Autodesk Inventor part; units mm, degrees
ref_plane "YZ Plane" through (0, 0, 0) normal (1, 0, 0) x (0, 1, 0)
ref_plane "XZ Plane" through (0, 0, 0) normal (0, 1, 0) x (-1, 0, 0)
ref_plane "XY Plane" through (0, 0, 0) normal (0, 0, 1) x (1, 0, 0)
sketch "Sketch1" plane through (0, 0, 0) normal (0, 0, 1) x (1, 0, 0)
  line L0 (17.5514, 0) -> (46.0756, 0)
  line L1 (46.0756, 0) -> (46.0756, 12.7)
  line L2 (46.0756, 12.7) -> (0, 12.7)
  line L3 (0, 12.7) -> (0, 0)
  line L4 (17.5514, 12.7) -> (17.5514, 0)
  line L5 (46.0756, 8.9662) -> (42.3672, 8.9662)
  line L6 (42.3672, 7.747) -> (42.3672, 0)
  line L7 (46.0756, 7.747) -> (42.3672, 7.747)
  line L8 (46.0756, 8.9662) -> (42.3672, 7.747)
  line L9 (0, 11.1252) -> (0, 12.7)
  line L10 (17.5514, 0) -> (23.85, 0)
  line L11 (0, -2.5) -> (0, 0)
  line L12 (0, 12.7) -> (38.0365, 12.7)
  line L13 (38.0365, 12.7) -> (38.0365, 14.2748)
  line L14 (38.0365, 14.2748) -> (0, 14.2748)
  line L15 (0, 14.2748) -> (0, 12.7)
  line L16 (17.5514, 12.7) -> (17.5514, 14.2748)
  line L17 (0, 0) -> (17.5514, 0)
  line L18 (0, 14.2748) -> (10.6426, 14.2748)
  line L19 (10.6426, 14.2748) -> (10.6426, 26.2128)
  line L20 (10.6426, 26.2128) -> (0, 26.2128)
  line L21 (0, 26.2128) -> (0, 14.2748)
  dimension "d1" = 12.7
  dimension "d3" = 3.7338
  dimension "d5" = 4.953
  dimension "d8" = 17.5514
  dimension "d9" = 42.3672
  dimension "d10" = 46.0756
  dimension "d11" = 1.5748
  dimension "d12" = 38.0365
  dimension "d23" = 11.938
  dimension "d24" = 10.6426
revolve "Revolution1" add sketch "Sketch1" angle 360 about axis through (0, 12.7, 0) along (0, -1, 0) contours L4 L2 L1 L8 L6 L0 | L17 L3 L2 L4 | L16 L14 L13 L2 | L2 L15 L14 L16 | L21 L20 L19 L14
sketch "Sketch2" plane through (0, 14.2748, 0) normal (0, 1, 0) x (1, 0, 0)
  circle A0 centre (0, 0) radius 30.1752
  point P0 (0, 30.1752)
  point P1 (0, -30.1752)
  dimension "d14" = 60.3504
hole "Hole1" at (0, 14.2748, -30.1752) at (0, 14.2748, 30.1752) direction (0, -1, 0) diameter 6.35 depth 7.62
fillet "Fillet1" radius 3.175 1 edges at (-42.3672, 0, 0)
sketch "Sketch3" plane through (0, 26.2128, 0) normal (0, 1, 0) x (1, 0, 0)
  point P0 (0, 0)
  point P1 (0, 0)
hole "Hole2" at (0, 26.2128, 0) direction (0, -1, 0) diameter 12.9794 end through all
chamfer "Chamfer1" distance 1.27 angle 45 1 edges at (0, 0, -6.4897)
chamfer "Chamfer2" distance 1.27 angle 45 1 edges at (-10.6426, 26.2128, 0)
properties part number "2016.06.09 ThorLabs Photodiode Adapter" material "Aluminum 6061"
CAD build for the part. Positions are in the model's coordinates, mm. A direction names the side the tool comes from. Give positions to 0.01 mm unless a question says otherwise; leave off trailing zeros. Write each question's results on one line, items separated by ' | '.
Q1. Probe probe 1 along Z at (x, y) = (0, 12.5); probe 2 along Z at (x, y) = (0, 16.25); probe 3 along Y at (x, z) = (2, 18). List the from-to ranges inside material, lowest first.
Geometry check:
probe 1: z = -46.08 to -33.35, -27 to -6.49, 6.49 to 27, 33.35 to 46.08 | probe 2: z = -10.64 to -6.49, 6.49 to 10.64 | probe 3: y = 0 to 14.27
Q2. Mould opens along X. For faces 3 (the face through (-0.954, 10.411, 33.204)), 4 (the face through (-9.18, 5.43, -41.36)), 5 (the face through (0, 6.655, 30)), 6 (the face through (7, 12.7, 38)) say: pulls with the +X half, pulls with the -X half, needs draft (parallel to the pull), parting line crosses it, or undercut.
Geometry check:
face 3: undercut | face 4: parting line crosses it | face 5: undercut | face 6: needs draft
Q3. Which spindle directions (+Z, -Z, +X, -X, +Y, -Y) get a long thin tool onto all of the face, cutting with end or side? Do faces 1 (the face through (0, 6.655, -30)), 2 (the face through (8, 0, 1)). Say none if no direction does.
Geometry check:
face 1: +Y | face 2: +Z, -Z, +X, -X, -Y
Q4. Flat gauge pins, fed straight in: P1, Ø5, axis at x = -1.5, z = 31, coming from the +Y side; P2, Ø8, axis at y = 3.5, z = 3, coming from the -X side; P3, Ø3, axis at x = -22, y = 12.5, coming from the +Z side; P4, Ø10.5, axis at x = 0, z = 0, coming from the -Y side. Where does each tip first touch, or does it go through?
Geometry check:
P1: stops at y = 14.27 | P2: stops at x = -42.37 | P3: stops at z = 41.26 | P4: passes through
